from build123d import *

# Parameters (mm, degrees)
SKETCH1_W           = 155
SKETCH1_H           = 70
BOSS_EXTRUDE1_DEPTH = 30
SKETCH2_W           = 70
SKETCH2_H           = 25
CUT_EXTRUDE1_DEPTH  = 71
SKETCH5_W           = 60
SKETCH5_H           = 25
CUT_EXTRUDE2_DEPTH  = 156
SKETCH6_W           = 80
SKETCH6_H           = 25
BOSS_EXTRUDE2_DEPTH = 5
SKETCH8_R           = 8
SKETCH8_R_2         = 2.5
CUT_EXTRUDE4_DEPTH  = 6
FILLET5_R           = 10
FILLET6_R           = 10


with BuildPart() as part:
    # Sketch1 → Boss-Extrude1 (new body)
    with BuildSketch(Plane(origin=(0, 0, 0), x_dir=(1, 0, 0), z_dir=(0, 1, 0))):
        with Locations((2.5, 0)):
            Rectangle(SKETCH1_W, SKETCH1_H)
    extrude(amount=BOSS_EXTRUDE1_DEPTH)

    # Sketch2 → Cut-Extrude1 (cut, through all)
    with BuildSketch(Plane.XY.offset(35)):
        with Locations((30, 17.5)):
            Rectangle(SKETCH2_W, SKETCH2_H)
    extrude(amount=-CUT_EXTRUDE1_DEPTH, mode=Mode.SUBTRACT)

    # Sketch5 → Cut-Extrude2 (cut, through all)
    with BuildSketch(Plane(origin=(80, 0, 0), x_dir=(0, 0, -1), z_dir=(1, 0, 0))):
        with Locations((0, 17.5)):
            Rectangle(SKETCH5_W, SKETCH5_H)
    extrude(amount=-CUT_EXTRUDE2_DEPTH, mode=Mode.SUBTRACT)

    # Sketch6 → Boss-Extrude2 (add)
    with BuildSketch(Plane(origin=(0, 0, 0), x_dir=(1, 0, 0), z_dir=(0, 1, 0))):
        with Locations((-1.578945933, -47.5)):
            Rectangle(SKETCH6_W, SKETCH6_H)
        with Locations((-1.578945933, 47.5)):
            Rectangle(SKETCH6_W, SKETCH6_H)
    extrude(amount=BOSS_EXTRUDE2_DEPTH)

    # Sketch8 → Cut-Extrude4 (cut, through all)
    with BuildSketch(Plane(origin=(0, 5, 0), x_dir=(1, 0, 0), z_dir=(0, 1, 0))):
        with Locations((5, 32.5)):
            Circle(SKETCH8_R)
        with Locations((5, -32.5)):
            Circle(SKETCH8_R)
        with Locations((-15, 52.5)):
            Circle(SKETCH8_R_2)
        with Locations((25, 12.5)):
            Circle(SKETCH8_R_2)
        with Locations((-15, -52.5)):
            Circle(SKETCH8_R_2)
        with Locations((25, -12.5)):
            Circle(SKETCH8_R_2)
    extrude(amount=-CUT_EXTRUDE4_DEPTH, mode=Mode.SUBTRACT)

    # Fillet5
    fillet5_edges = [part.edges().sort_by_distance(p)[0] for p in [
        (38.421054067, 2.5, 60),
    ]]
    fillet(fillet5_edges, radius=FILLET5_R)

    # Fillet6
    fillet6_edges = [part.edges().sort_by_distance(p)[0] for p in [
        (-41.578945933, 2.5, -60),
        (38.421054067, 2.5, -60),
        (-41.578945933, 2.5, 60),
    ]]
    fillet(fillet6_edges, radius=FILLET6_R)


solid = part.part
Geometry: final body of the model. Coordinates: model frame, mm. A direction names the side the tool comes from. Give positions to 0.01 mm unless a question says otherwise; leave off trailing zeros. Order: outer loops, then holes, each group sorted by start corner. A loop starts at its lowest first (then second) coordinate and runs counter-clockwise, first axis right, second up. Notation, with made-up numbers: (55, 13) - (81, 13) arc R23 cw to (81, 25) - close; hole circle Ø2 at (-18, 15). An arc over 180 degrees is marked (long way). Use CSV: the item, a comma, the result in double quotes.
1. Access query for faces 4 (the face through (38.421, 2, 43)), 5 (the face through (-41.579, 2, 43)), 6 (the face through (65, 17, 33)), 7 (the face through (38.421, 2, -42)). Directions: +Z, -Z, +X, -X, +Y, -Y. A direction counts if a zero-diameter tool reaches every point of the face in a straight line with its end or side. Return the directions, or none.
Answers below:
face 4,"+Z, +X, +Y, -Y"
face 5,"+Z, -X, +Y, -Y"
face 6,"+Z, -Z, +Y"
face 7,"-Z, +X, +Y, -Y"
2. Section query B-B (z = -32.5). Output: boundary loops of the cut face in (x, y), plus the area to 3 significant figures.
Answers below:
outline,"(-75, 0) - (-3, 0) - (-3, 5) - (-5, 5) - (-5, 30) - (-75, 30) - close; (13, 0) - (80, 0) - (80, 30) - (65, 30) - (65, 5) - (13, 5) - close"
area,"2,820 mm2"
3. Contact query for flat-ended pins moving along their axis: pin 1 (12 mm diameter, centred on x = 24, z = 36.5, fed in from +Y); pin 2 (16.5 mm diameter, centred on x = 75, y = 23.5, fed in from -Z); pin 3 (6 mm diameter, centred on y = 24.5, z = -26.5, fed in from -X) (3 decimals); pin 4 (5 mm diameter, centred on x = -43.5, y = 8.5, fed in from +Z). Output: stop coordinate, or through.
Answers below:
pin 1,"y = 5"
pin 2,"z = -35"
pin 3,"through"
pin 4,"z = 35"
4. Section query C-C (y = 18.5). Output: boundary loops of the cut face in (x, z).
Answers below:
outline,"(-75, -35) - (-5, -35) - (-5, -30) - (-75, -30) - close; (-75, 30) - (-5, 30) - (-5, 35) - (-75, 35) - close; (65, -35) - (80, -35) - (80, -30) - (65, -30) - close; (65, 30) - (80, 30) - (80, 35) - (65, 35) - close"
5. Material intervals for line 1 along Z through (x, y) = (5, 4.05); line 2 along Z through (x, y) = (-15, 1.35); line 3 along Z through (x, y) = (52.5, 3), sorted ascending. Write a range as from..to.
Answers below:
line 1,"-60..-40.5, -24.5..24.5, 40.5..60"
line 2,"-60..-55, -50..50, 55..60"
line 3,"-35..35"
6. Mould query, pull axis X, two halves, no side actions, for faces 1 (the face through (1, 0, -1)), 2 (the face through (-38.73, 2.54, -56.99)), 3 (the face through (65, 17, -32)). Classes: +X half, -X half, draft (parallel to the pull), parting line (faces both ways), or undercut.
Answers below:
face 1,"draft"
face 2,"-X half"
face 3,"undercut"
7. Section query A-A (x = 5). Output: boundary loops of the cut face in (y, z).
Answers below:
outline,"(0, -60) - (5, -60) - (5, -40.5) - (0, -40.5) - close; (0, -24.5) - (5, -24.5) - (5, 24.5) - (0, 24.5) - close; (0, 40.5) - (5, 40.5) - (5, 60) - (0, 60) - close"
8. Section query D-D (x = -53). Output: boundary loops of the cut face in (y, z).
Answers below:
outline,"(0, -35) - (30, -35) - (30, -30) - (5, -30) - (5, 30) - (30, 30) - (30, 35) - (0, 35) - close"
